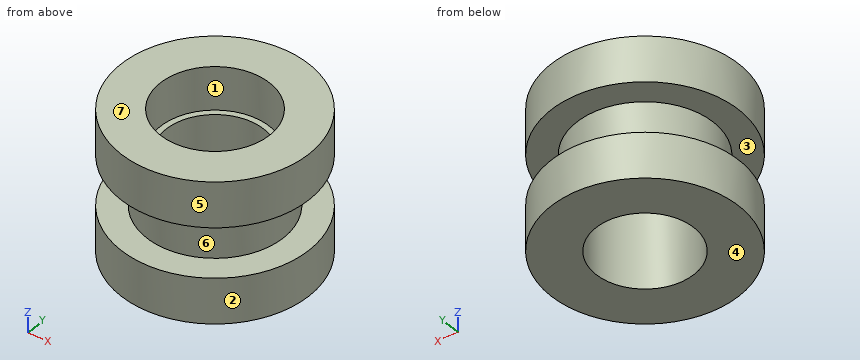
from build123d import *

# Parameters (mm, degrees)
F0_R     = 4.125
F0_R_2   = 3
F1_DEPTH = 2
F0_R_3   = 2.15
F2_DEPTH = 6.2
F3_R     = 4.125
F3_R_2   = 3
F4_DEPTH = 2
F3_R_3   = 2.4
F3_R_4   = 2.15
F5_DEPTH = 1.9


with BuildPart() as f1:
    # F0 (on Top) → F1 (new body)
    with BuildSketch(Plane.XY):
        Circle(F0_R)
        Circle(F0_R_2, mode=Mode.SUBTRACT)
    extrude(amount=F1_DEPTH)

    # F0 (on Top) → F2 (join)
    with BuildSketch(Plane.XY):
        Circle(F0_R_2)
        Circle(F0_R_3, mode=Mode.SUBTRACT)
    extrude(amount=F2_DEPTH)

    # F3 (on face) → F4 (join)
    with BuildSketch(Plane.XY.offset(6.2)):
        Circle(F3_R)
        Circle(F3_R_2, mode=Mode.SUBTRACT)
    extrude(amount=-F4_DEPTH)

    # F3 (on face) → F5 (cut)
    with BuildSketch(Plane.XY.offset(6.2)):
        Circle(F3_R_3)
        Circle(F3_R_4, mode=Mode.SUBTRACT)
        Circle(F3_R_4)
    extrude(amount=-F5_DEPTH, mode=Mode.SUBTRACT)


solid = f1.part
Could you check a few things on this model? Use its own coordinates, in mm. Face numbers are marked on the shaded views. A direction names the side the tool comes from. Give positions to 0.01 mm unless a question says otherwise; leave off trailing zeros. Order: outer loops, then holes, each group sorted by start corner. A loop starts at its lowest first (then second) coordinate and runs counter-clockwise, first axis right, second up. Notation, with made-up numbers: (52, -37) -> (67, -37) arc R11 cw to (67, -25) -> close; hole circle Ø5 at (-22, 56). An arc over 180 degrees is marked (long way). Return JSON: item names as keys, results as strings.
1. For pin 1 Ø2 at (y, z) = (-3, 4) entering from +X; pin 2 Ø1.5 at (x, z) = (3, 4) entering from -Y, each with a flat end and sliding along its axis, tell me the tip position at first contact or that it passes through.
Answer list:
{"pin 1": "stops at x = 3.6", "pin 2": "stops at y = -3.44"}
2. Imagine slicing it at D-D on y = 3.5. List the corners of the cut face in (x, z) for me, then the cut area to 3 significant figures.
Answer list:
{"outline": "(-2.18, 0) -> (2.18, 0) -> (2.18, 2) -> (-2.18, 2) -> close; (-2.18, 4.2) -> (2.18, 4.2) -> (2.18, 6.2) -> (-2.18, 6.2) -> close", "area": "17.5 mm2"}
3. On a 3-axis mill with a long thin cutter (end or side, diameter ignored), from which of +Z, -Z, +X, -X, +Y, -Y can I reach the whole of each face in a straight line? I mean the marked faces 1, 2 and 3. Say none if no direction works.
Answer list:
{"face 1": "+Z", "face 2": "+Z, -Z", "face 3": "none"}
4. Imagine slicing it at A-A on y = 0. List the corners of the cut face in (x, z) for me (3 decimals), then the cut area to 3 significant figures.
Answer list:
{"outline": "(-4.125, 0) -> (-2.15, 0) -> (-2.15, 4.3) -> (-2.4, 4.3) -> (-2.4, 6.2) -> (-4.125, 6.2) -> (-4.125, 4.2) -> (-3, 4.2) -> (-3, 2) -> (-4.125, 2) -> close; (2.15, 0) -> (4.125, 0) -> (4.125, 2) -> (3, 2) -> (3, 4.2) -> (4.125, 4.2) -> (4.125, 6.2) -> (2.4, 6.2) -> (2.4, 4.3) -> (2.15, 4.3) -> close", "area": "18.6 mm2"}
5. I need wall thicknesses on line 1 (Z direction, x = -1, y = -3.75); line 2 (Y direction, x = 0, z = 5.25) (3 decimals); line 3 (X direction, y = 1.5, z = 4.25). Which ranges of each line are inside material? Lowest first, please. Write a range as from..to.
Answer list:
{"line 1": "z = 0..2, 4.2..6.2", "line 2": "y = -4.125..-2.4, 2.4..4.125", "line 3": "x = -3.84..-1.54, 1.54..3.84"}
6. Thinking about a two-plate mould opening in Z: for the marked faces 4, 5, 6 and 7, which applies, pulls with the +Z half, pulls with the -Z half, needs draft (parallel to the pull), parting line crosses it, or undercut?
Answer list:
{"face 4": "pulls with the -Z half", "face 5": "needs draft", "face 6": "undercut", "face 7": "pulls with the +Z half"}
7. Imagine slicing it at C-C on z = 3.5. List the corners of the cut face in (x, y) for me.
Answer list:
{"outline": "circle Ø6 at (0, 0); hole circle Ø4.3 at (0, 0)"}
